Check sheet for the modelled part. Datum: model origin and axes. Units: mm. Face numbers are marked on the shaded views. Give positions to 0.01 mm unless a question says otherwise; leave off trailing zeros. Order: outer loops, then holes, each group sorted by start corner. A loop starts at its lowest first (then second) coordinate and runs counter-clockwise, first axis right, second up.
```python
from build123d import *

# Parameters (mm, degrees)
SKETCH1_R           = 19
SKETCH1_R_2         = 17
BOSS_EXTRUDE1_DEPTH = 125
SKETCH4_R           = 4
CUT_EXTRUDE3_DEPTH  = 41


with BuildPart() as part:
    # Sketch1 → Boss-Extrude1 (new body, symmetric)
    with BuildSketch(Plane.XY):
        Circle(SKETCH1_R)
        Circle(SKETCH1_R_2, mode=Mode.SUBTRACT)
    extrude(amount=BOSS_EXTRUDE1_DEPTH, both=True)

    # Sketch4 → Cut-Extrude3 (cut, through all)
    with BuildSketch(Plane(origin=(0, 21, 0), x_dir=(1, 0, 0), z_dir=(0, 1, 0))):
        with Locations((0, -100)):
            Circle(SKETCH4_R)
    cut_extrude3 = extrude(amount=-CUT_EXTRUDE3_DEPTH, mode=Mode.SUBTRACT)

    # Mirror1: Cut-Extrude3 across plane
    add(cut_extrude3.mirror(Plane.XY), mode=Mode.SUBTRACT)


solid = part.part
```
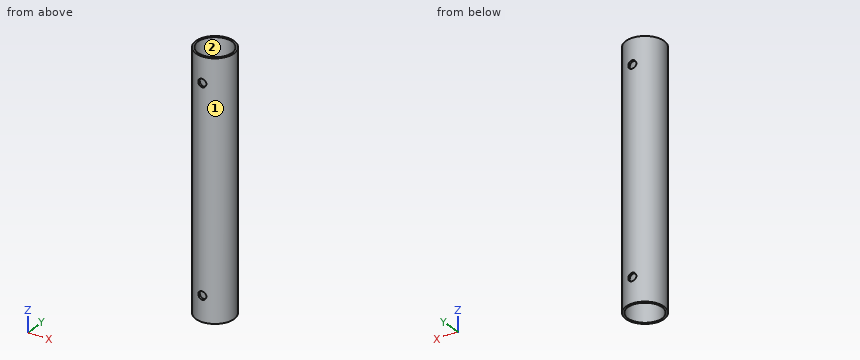
Q1. Go/stop test with flat-tipped pins: P1, Ø8, axis at x = 15, z = -23.5, coming from the -Y side; P2, Ø1.5, axis at y = -7, z = 17, coming from the -X side; P3, Ø5, axis at x = 7.5, z = 54.5, coming from the -Y side. Record where each tip stops, or that it passes through.
Q2. Draft check along X on the marked faces 1 and 2. Enter one of: pulls with the +X half, pulls with the -X half, needs draft (parallel to the pull), parting line crosses it, or undercut.
Q3. Sectioned sample at B-B, the plane x = -9. Record the cut outline in (y, z).
Q4. Sectioned sample at D-D, the plane z = -37. Record the cut outline in (x, y), plus the area to 3 significant figures.
Q5. Sectioned sample at A-A, the plane y = 0. Record the cut outline in (x, z), plus the area to 3 significant figures.
Q6. Sectioned sample at C-C, the plane x = 0. Record the cut outline in (y, z), plus the area to 3 significant figures.
Q7. Material ranges on line 1 (Z direction, x = 0, y = -17.5); line 2 (X direction, y = -1, z = -71); line 3 (Y direction, x = 0, z = -44), recorded low to high.
Filled in:
1. P1: stops at y = -15.49
1. P2: stops at x = -17.94
1. P3: stops at y = -18.33
2. face 1: parting line crosses it
2. face 2: undercut
3. outline: (-16.73, -125) - (-14.42, -125) - (-14.42, 125) - (-16.73, 125) - close; (14.42, -125) - (16.73, -125) - (16.73, 125) - (14.42, 125) - close
4. outline: circle Ø38 at (0, 0); hole circle Ø34 at (0, 0)
4. area: 226 mm2
5. outline: (-19, -125) - (-17, -125) - (-17, 125) - (-19, 125) - close; (17, -125) - (19, -125) - (19, 125) - (17, 125) - close
5. area: 1,000 mm2
6. outline: (-19, -125) - (-17, -125) - (-17, -104) - (-19, -104) - close; (-19, -96) - (-17, -96) - (-17, 96) - (-19, 96) - close; (-19, 104) - (-17, 104) - (-17, 125) - (-19, 125) - close; (17, -125) - (19, -125) - (19, -104) - (17, -104) - close; (17, -96) - (19, -96) - (19, 96) - (17, 96) - close; (17, 104) - (19, 104) - (19, 125) - (17, 125) - close
6. area: 936 mm2
7. line 1: z = -125 to -104, -96 to 96, 104 to 125
7. line 2: x = -18.97 to -16.97, 16.97 to 18.97
7. line 3: y = -19 to -17, 17 to 19
